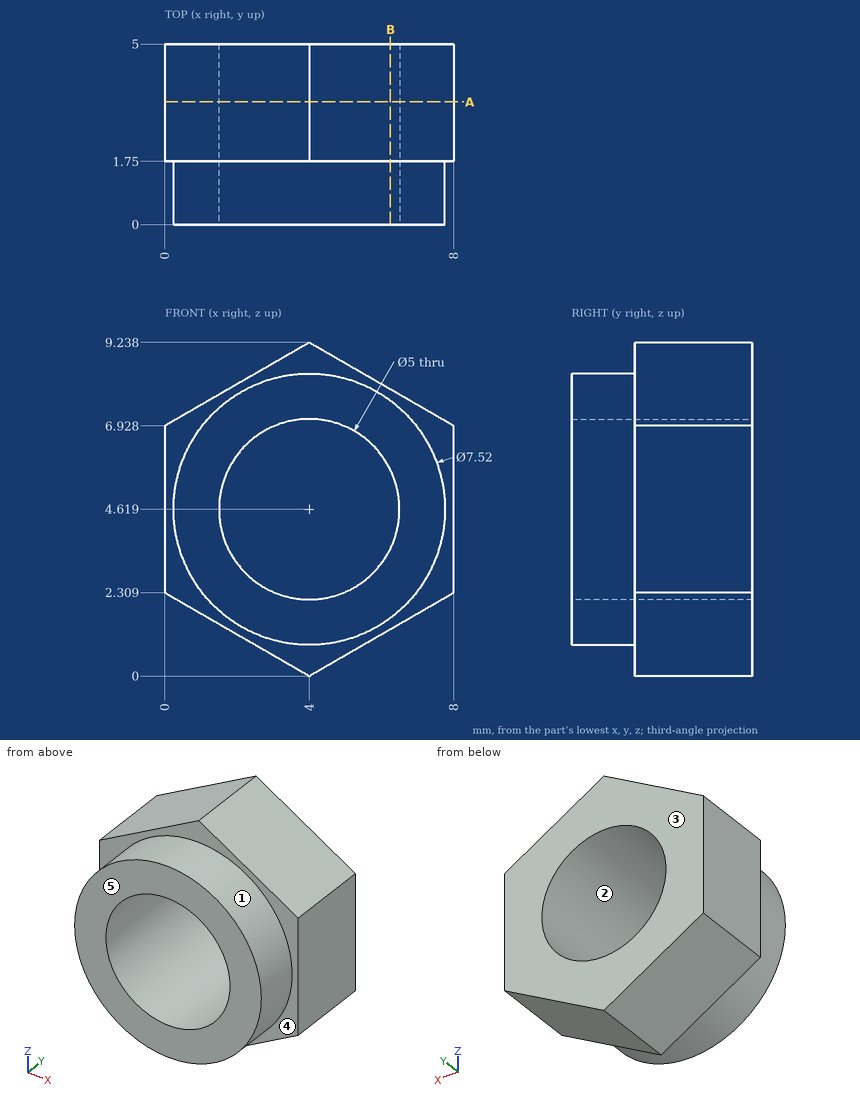
The drawing under review shows one solid part. Ordinate dimensions are in mm from its lowest x, y, z. A direction names the side the tool comes from. Coordinates: 2 decimals unless noted, no trailing zeros. Write each loop counter-clockwise with the first axis right and the second up, starting at its lowest first coordinate (ties: lowest second). Pieces come first, ordered by that corner, then holes. Notation, with made-up numbers: (11.5, -4) -> (65.5, -4) arc R21 ccw to (65.5, 27) -> close; hole circle Ø2 at (73, -1.5). An arc over 180 degrees is marked (long way). Write each question's results on one line, items separated by ' | '. Start each with the question number.
1) Consider section A-A (y = 3.4). Write out the cut boundary in (x, z), plus the area to 3 significant figures.
2) For the marked faces 4 and 5, list the 3-axis set-ups (+Z, -Z, +X, -X, +Y, -Y) from which the entire face can be reached by the end or side of a thin tool; tool diameter is ignored.
3) The part is to be moulded in two halves that separate along X. For the marked faces 1, 2 and 3, say which applies: +X half, -X half, draft (parallel to the pull), parting line (faces both ways), or undercut.
4) Wall thickness on L1, parallel to X at y = 0.5, z = 4.5; L2, parallel to X at y = 1, z = 2.5 (1 decimal); L3, parallel to Z at x = 3, y = 0.65 (1 decimal): over which ranges is each line inside the solid? List them lowest first. Write a range as [from, to].
5) Consider section B-B (x = 6.25). Write out the cut boundary in (y, z), plus the area to 3 significant figures.
6) Insertion check: pin 1 (3 mm diameter, centred on x = 4, z = 4.62, fed in from +Y). The pin has a flat end and moves straight along its axis. Give the tip position at first contact, or say it passes through.
Geometry says:
1) outline: (0, 2.31) -> (4, 0) -> (8, 2.31) -> (8, 6.93) -> (4, 9.24) -> (0, 6.93) -> close; hole circle Ø5 at (4, 4.62) | area: 35.8 mm^2
2) face 4: -Y | face 5: +Z, -Z, +X, -X, -Y
3) face 1: parting line | face 2: undercut | face 3: draft
4) L1: [0.24, 1.5], [6.5, 7.76] | L2: [0.9, 2.7], [5.3, 7.1] | L3: [1, 2.3], [6.9, 8.2]
5) outline: (0, 1.61) -> (1.75, 1.61) -> (1.75, 1.3) -> (5, 1.3) -> (5, 3.53) -> (0, 3.53) -> close; (0, 5.71) -> (5, 5.71) -> (5, 7.94) -> (1.75, 7.94) -> (1.75, 7.63) -> (0, 7.63) -> close | area: 21.2 mm^2
6) pin 1: through
